Check sheet for the modelled part. Datum: model origin and axes. Units: mm. Face numbers are marked on the shaded views. A direction names the side the tool comes from. Coordinates: 2 decimals unless noted, no trailing zeros. Loops run counter-clockwise (first coordinate to the right, second up) from the corner with the lowest first, then second, coordinate; pieces in that order, holes last. Notation, with made-up numbers: (77, 71.25) -> (120, 71.25) arc R29 cw to (120, 102.25) -> close; hole circle Ø4 at (42, 44.5). An arc over 180 degrees is marked (long way). Use CSV: the item, a comma, the result in double quotes.
```python
from build123d import *

# Parameters (mm, degrees)
EXTRUDE_1_DEPTH      = 4
EXTRUDE_START        = -2
SKETCH_2_3_R         = 0.625
EXTRUDE_2_DEPTH      = 1
EXTRUDE_3_DEPTH      = 1.5
EXTRUDE_3_DEPTH_BACK = 4.02
SKETCH_4_R           = 0.45
SKETCH_5_R           = 1.5
EXTRUDE_4_DEPTH      = 0.02


with BuildPart() as part:
    # 草图2 → 凸台-拉伸1 (new body)
    with BuildSketch(Plane.XY):
        with BuildLine():
            Line((-12.1, 2.25), (12.1, 2.25))
            ThreePointArc((12.1, 2.25), (14.35, 0), (12.1, -2.25))
            Line((12.1, -2.25), (-12.1, -2.25))
            ThreePointArc((-12.1, -2.25), (-14.35, 0), (-12.1, 2.25))
        make_face()
    extrude(amount=-EXTRUDE_1_DEPTH)

    # 草图2<3> → 凸台-拉伸2 (add)
    with BuildSketch(Plane.XY.offset(EXTRUDE_START)):
        with BuildLine():
            Line((-15.37, 2.25), (15.37, 2.25))
            ThreePointArc((15.37, 2.25), (17.62, 0), (15.37, -2.25))
            Line((15.37, -2.25), (-15.37, -2.25))
            ThreePointArc((-15.37, -2.25), (-17.62, 0), (-15.37, 2.25))
        make_face()
        with Locations((-15.87, 0)):
            Circle(SKETCH_2_3_R, mode=Mode.SUBTRACT)
        with Locations((15.87, 0)):
            Circle(SKETCH_2_3_R, mode=Mode.SUBTRACT)
    extrude(amount=-EXTRUDE_2_DEPTH)

    # 草图4 → 凸台-拉伸3 (add, two sides: drawn at the far end of the back side and taken through both)
    with BuildSketch(Plane(origin=(0, 0, -4), x_dir=(-1, 0, 0), z_dir=(0, 0, -1)).offset(-EXTRUDE_3_DEPTH_BACK)):
        with Locations(Location((-8.89, 0, 0), (0, 0, 180))):
            Circle(SKETCH_4_R)
        with Locations(Location((-6.35, 0, 0), (0, 0, 180))):
            Circle(SKETCH_4_R)
        with Locations(Location((-3.81, 0, 0), (0, 0, 180))):
            Circle(SKETCH_4_R)
        with Locations(Location((-1.27, 0, 0), (0, 0, 180))):
            Circle(SKETCH_4_R)
        with Locations(Location((1.27, 0, 0), (0, 0, 180))):
            Circle(SKETCH_4_R)
        with Locations(Location((3.81, 0, 0), (0, 0, 180))):
            Circle(SKETCH_4_R)
        with Locations(Location((6.35, 0, 0), (0, 0, 180))):
            Circle(SKETCH_4_R)
        with Locations(Location((8.89, 0, 0), (0, 0, 180))):
            Circle(SKETCH_4_R)
    extrude(amount=EXTRUDE_3_DEPTH + EXTRUDE_3_DEPTH_BACK)

    # 草图5 → 凸台-拉伸4 (add)
    with BuildSketch(Plane.XY):
        with Locations(Location((-12.1, 0, 0), (0, 0, 180))):
            Circle(SKETCH_5_R)
        with Locations(Location((12.1, 0, 0), (0, 0, 180))):
            Circle(SKETCH_5_R)
    extrude(amount=EXTRUDE_4_DEPTH)


solid = part.part
```
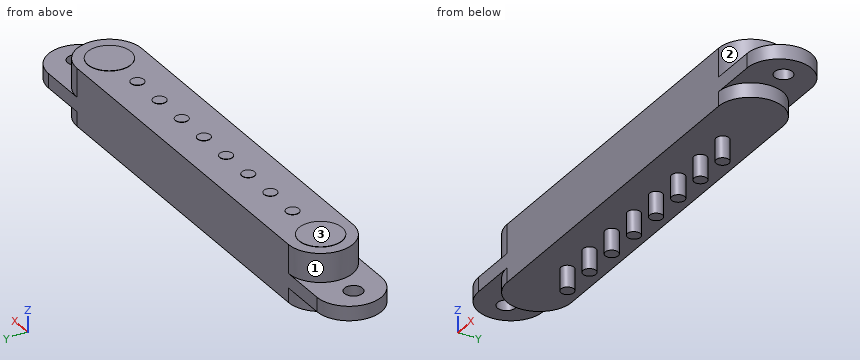
1) Access from +Z, -Z, +X, -X, +Y, -Y to the whole of each face (thin tool, end or side, straight path). Record for the marked faces 1, 2 and 3.
Answer below:
face 1,"+Z, -X"
face 2,"+Z, +X"
face 3,"+Z, +X, -X, +Y, -Y"
2) Cross-section at D-D on x = -15.87. Record the boundary of the cut face in (y, z) (3 decimals), and give its area (3 significant figures).
Answer below:
outline,"(-2.194, -3) -> (-0.625, -3) -> (-0.625, -2) -> (-2.194, -2) -> close; (0.625, -3) -> (2.194, -3) -> (2.194, -2) -> (0.625, -2) -> close"
area,"3.14 mm²"
3) Go/stop test with flat-tipped pins: pin 1 Ø1.6 at (x, y) = (-15.87, 0) entering from -Z; pin 2 Ø2 at (x, y) = (-15, 0) entering from -Z; pin 3 Ø1 at (y, z) = (1, -0.5) entering from +X; pin 4 Ø2 at (x, y) = (-4, -0.5) entering from -Z. Record where each tip stops, or that it passes through.
Answer below:
pin 1,"stops at z = -3"
pin 2,"stops at z = -4"
pin 3,"stops at x = 14.29"
pin 4,"stops at z = -5.5"
4) Cross-section at C-C on y = 0. Give the number of separate pieces and of enclosed holes in the cut face, and give its area (3 significant figures).
Answer below:
separate pieces,"3"
enclosed holes,"0"
area,"130 mm²"
5) Thickness scan on line 1 along Z through (x, y) = (-8, 1.55); line 2 along Y through (x, z) = (15.87, -2.45) (3 decimals); line 3 along X through (y, z) = (0.4, -0.3). Record the ranges inside material, lowest first. Write a range as from..to.
Answer below:
line 1,"z = -4..0"
line 2,"y = -2.194..-0.625, 0.625..2.194"
line 3,"x = -14.31..14.31"
6) Cross-section at A-A on z = -4.7. Record the boundary of the cut face in (x, y).
Answer below:
outline,"circle Ø0.9 at (-8.89, 0); circle Ø0.9 at (-6.35, 0); circle Ø0.9 at (-3.81, 0); circle Ø0.9 at (-1.27, 0); circle Ø0.9 at (1.27, 0); circle Ø0.9 at (3.81, 0); circle Ø0.9 at (6.35, 0); circle Ø0.9 at (8.89, 0)"
